Read the model definition and answer for the solid it produces. Units are mm, in the model's axes. Coordinates: 2 decimals unless noted, no trailing zeros. Write each loop counter-clockwise with the first axis right and the second up, starting at its lowest first coordinate (ties: lowest second). Pieces come first, ordered by that corner, then holes. Notation, with made-up numbers: (52, 6) -> (72, 6) arc R27 cw to (72, 23) -> close; hole circle Ø11 at (32.5, 82). An arc over 180 degrees is marked (long way). One line per item, written item: value. Start each with the question number.
1. Find section A-A, the plane y = 0. Write down the section's boundary in (x, z).
2. Given P1, Ø3, axis at y = 0, z = 10, coming from the -X side, flat-ended and moving along its own axis, determine where the tip first touches the part or whether it passes through.
3. Consider line 1 along Z through (x, y) = (-4.35, 0); line 2 along Z through (x, y) = (0, -4.5); line 3 along X through (y, z) = (1.75, 141). Determine where each line is inside the solid, lowest interval first.
4. Find section B-B, the plane x = 0. Write down the section's boundary in (y, z).
5. Find section C-C, the plane z = 142. Write down the section's boundary in (x, y).
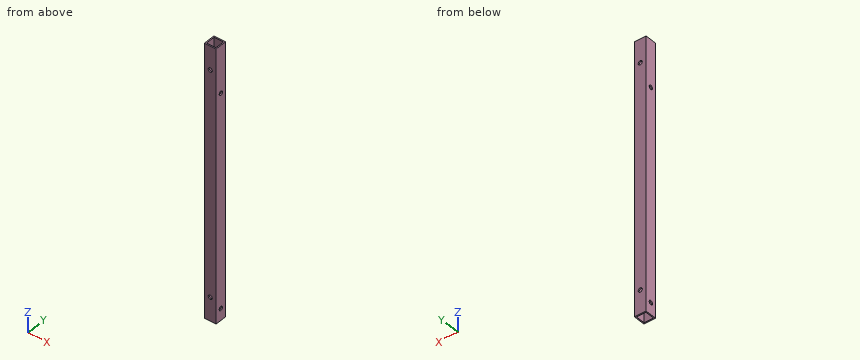
Autodesk Inventor part; units mm, degrees
ref_plane "YZ Plane" through (0, 0, 0) normal (1, 0, 0) x (0, 1, 0)
ref_plane "XZ Plane" through (0, 0, 0) normal (0, 1, 0) x (-1, 0, 0)
ref_plane "XY Plane" through (0, 0, 0) normal (0, 0, 1) x (1, 0, 0)
sketch "スケッチ1" plane through (0, 0, 0) normal (0, 0, 1) x (1, 0, 0)
  line L0 (5, -5) -> (-5, -5)
  line L1 (-5, -5) -> (-5, 5)
  line L2 (-5, 5) -> (5, 5)
  line L3 (5, 5) -> (5, -5)
  line L4 (5, -5) -> (-5, 5) construction
  line L5 (-5, -5) -> (5, 5) construction
  line L6 (4, 4) -> (-4, 4)
  line L7 (-4, 4) -> (-4, -4)
  line L8 (-4, -4) -> (4, -4)
  line L9 (4, -4) -> (4, 4)
  point P0 (0, 0)
  dimension "d0" = 10
  dimension "d1" = 10
  dimension "d2" = 1
extrude "押し出し1" add sketch "スケッチ1" along normal blind 230
sketch "スケッチ2" plane through (5, -5, 0) normal (1, 0, 0) x (0, 0, -1)
  line L0 (0, 5) -> (-228.6606, 5)
  line L1 (0, 0) -> (0, 10)
  point P0 (-190, 5)
  point P1 (-10, 5)
  dimension "d5" = 180
  dimension "d6" = 10
hole "穴1" at (5, 0, 190) at (5, 0, 10) direction (-1, 0, 0) diameter 3.5 end through all
sketch "スケッチ3" plane through (-5, 5, 0) normal (0, 1, 0) x (1, 0, 0)
  line L0 (5, 0) -> (5, -230)
  line L1 (9, -230) -> (1, -230)
  line L2 (10, 0) -> (0, 0)
  point P0 (5, -210)
  point P1 (5, -20)
  dimension "d14" = 20
  dimension "d15" = 190
hole "穴2" at (0, 5, 210) at (0, 5, 20) direction (0, -1, 0) diameter 3.5 end through all
properties part number "small_kaku_1010_bridge"
Answer block:
1. outline: (-5, 0) -> (-4, 0) -> (-4, 8.25) -> (-5, 8.25) -> close; (-5, 11.75) -> (-4, 11.75) -> (-4, 188.25) -> (-5, 188.25) -> close; (-5, 191.75) -> (-4, 191.75) -> (-4, 230) -> (-5, 230) -> close; (4, 0) -> (5, 0) -> (5, 8.25) -> (4, 8.25) -> close; (4, 11.75) -> (5, 11.75) -> (5, 188.25) -> (4, 188.25) -> close; (4, 191.75) -> (5, 191.75) -> (5, 230) -> (4, 230) -> close
2. P1: passes through
3. line 1: z = 0 to 8.25, 11.75 to 188.25, 191.75 to 230
3. line 2: z = 0 to 18.25, 21.75 to 208.25, 211.75 to 230
3. line 3: x = -5 to -4, 4 to 5
4. outline: (-5, 0) -> (-4, 0) -> (-4, 18.25) -> (-5, 18.25) -> close; (-5, 21.75) -> (-4, 21.75) -> (-4, 208.25) -> (-5, 208.25) -> close; (-5, 211.75) -> (-4, 211.75) -> (-4, 230) -> (-5, 230) -> close; (4, 0) -> (5, 0) -> (5, 18.25) -> (4, 18.25) -> close; (4, 21.75) -> (5, 21.75) -> (5, 208.25) -> (4, 208.25) -> close; (4, 211.75) -> (5, 211.75) -> (5, 230) -> (4, 230) -> close
5. outline: (-5, -5) -> (5, -5) -> (5, 5) -> (-5, 5) -> close; hole (-4, -4) -> (4, -4) -> (4, 4) -> (-4, 4) -> close
